Study the drawing (mm; zero at the part's minimum x, y, z) and answer. Give positions to 0.01 mm unless a question says otherwise; leave off trailing zeros. Order: outer loops, then holes, each group sorted by start corner. A loop starts at its lowest first (then second) coordinate and runs counter-clockwise, first axis right, second up.
Item 1: A cutting plane is placed at A-A (x = 10.5). Write down the section's boundary in (y, z).
Item 2: A cutting plane is placed at B-B (z = 12.5). Write down the section's boundary in (x, y), plus the area to 3 significant figures.
Item 3: Given pin 1 Ø1.5 at (x, z) = (18, 16.5) entering from -Y; pin 2 Ø8 at (x, y) = (16, 5) entering from -Z; pin 3 Ø6 at (x, y) = (6.5, 8) entering from +Z, each flat-ended and moving along its own axis, determine where each tip first touches the part or whether it passes through.
Item 4: A cutting plane is placed at C-C (y = 5.5). Write down the section's boundary in (x, z), plus the area to 3 significant figures.
Item 5: Find the intervals of material crossed by line 1 along X through (y, z) = (8.5, 14); line 2 along X through (y, z) = (18.75, 3.75); line 3 along Z through (x, y) = (5, 9.5), in increasing order.
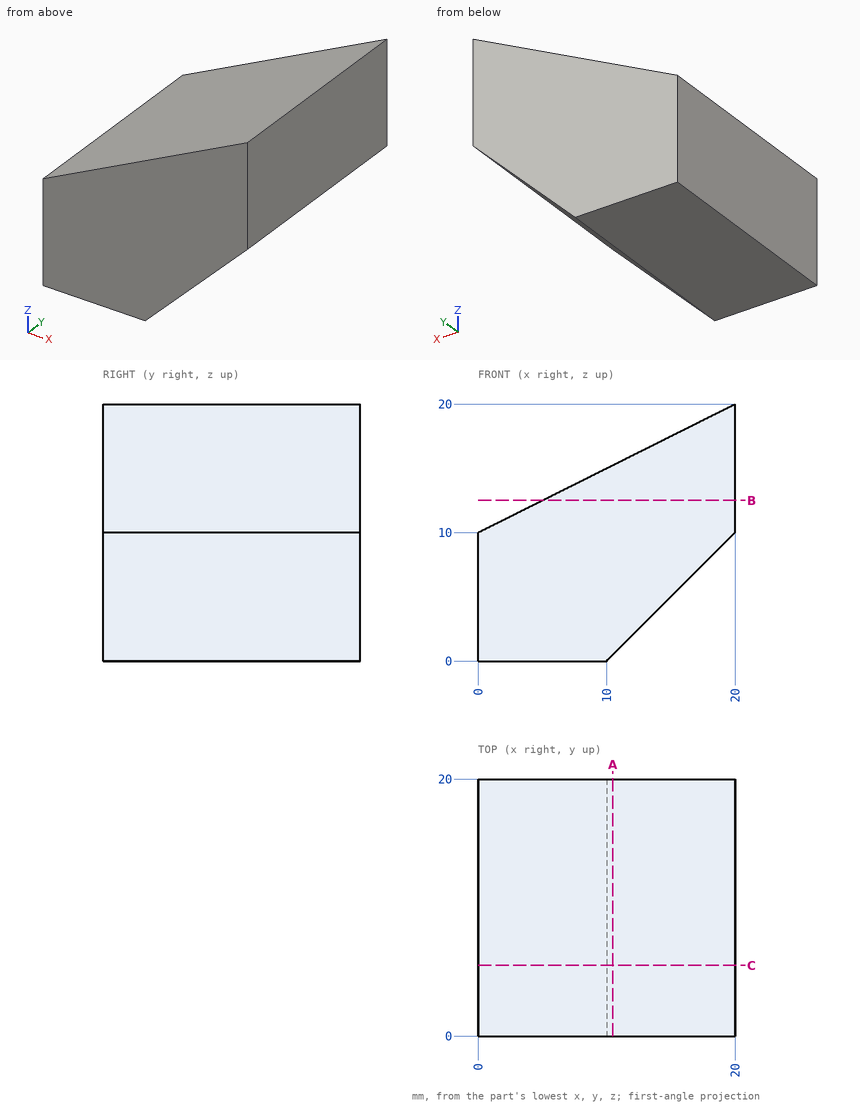
Response values:
1. outline: (0, 0.5) - (20, 0.5) - (20, 15.25) - (0, 15.25) - close
2. outline: (5, 0) - (20, 0) - (20, 20) - (5, 20) - close
2. area: 300 mm2
3. pin 1: stops at y = 0
3. pin 2: stops at z = 2
3. pin 3: stops at z = 14.75
4. outline: (0, 0) - (10, 0) - (20, 10) - (20, 20) - (0, 10) - close
4. area: 250 mm2
5. line 1: x = 8 to 20
5. line 2: x = 0 to 13.75
5. line 3: z = 0 to 12.5
